Autodesk Inventor part; units mm, degrees
ref_plane "YZ Plane" through (0, 0, 0) normal (1, 0, 0) x (0, 1, 0)
ref_plane "XZ Plane" through (0, 0, 0) normal (0, 1, 0) x (-1, 0, 0)
ref_plane "XY Plane" through (0, 0, 0) normal (0, 0, 1) x (1, 0, 0)
sketch "Sketch1" plane through (0, 0, 0) normal (0, 0, 1) x (1, 0, 0)
  line L0 (0, 0) -> (30, 0) construction
  line L1 (30, 0) -> (30, 30) construction
  line L2 (30, 30) -> (0, 30) construction
  line L3 (0, 11.9722) -> (0, 0) construction
  circle A0 centre (0, 0) radius 30 construction
  circle A1 centre (30, 30) radius 30 construction
  circle A2 centre (30, 30) radius 35
  arc A3 (29.5798, 5.0035) -> (5.0035, 29.5798) centre (30, 30) ccw
  arc A4 (29.5798, 5.0035) -> (5.0035, 29.5798) centre (0, 0) ccw
  line L4 (30, 30) -> (0, 0) construction
  circle A5 centre (30, 30) radius 4
  circle A6 centre (8.7868, 8.7868) radius 3
  dimension "d3" = 60
  dimension "d4" = 70
  dimension "d0" = 30
  dimension "d1" = 30
  dimension "d2" = 60
  dimension "d5" = 50
  dimension "d6" = 8
  dimension "d7" = 6
extrude "Extrusion1" add sketch "Sketch1" along normal blind 5 contours A4 A3 | A6
extrude "Extrusion2" add sketch "Sketch1" against normal blind 5 contours A2 | A4 A3 | A6
properties part number "Geneva_driver"
The listing builds one solid part. Answer for the finished solid, in the listing's coordinates (mm). A direction names the side the tool comes from. Give positions to 0.01 mm unless a question says otherwise; leave off trailing zeros. Order: outer loops, then holes, each group sorted by start corner. A loop starts at its lowest first (then second) coordinate and runs counter-clockwise, first axis right, second up. Notation, with made-up numbers: (84, -9.5) - (141, -9.5) arc R20 ccw to (141, -2.5) - close; hole circle Ø1 at (60, 19). An arc over 180 degrees is marked (long way). Answer in a Markdown table with one row per item. Add a question column.
Q1. The part is cut by section A-A (z = -1). Determine the outline of the cut face in (x, y), then the cut area to 3 significant figures.
Q2. Find the intervals of material crossed by line 1 along Y through (x, z) = (30, -2); line 2 along Z through (x, y) = (11.5, 55.5); line 3 along Y through (x, z) = (30, 0.25), in increasing order. Write a range as [from, to].
Q3. Which of the six approach directions +Z, -Z, +X, -X, +Y, -Y give full straight-line access (tool end or side, diameter ignored) to faces 4 (the cylindrical face through (21.029, 21.396, 2.465)), 5 (the cylindrical face through (29.479, 26.034, -0.07))?
Q4. The part is cut by section C-C (y = 17). Determine the outline of the cut face in (x, z).
Q5. Given P1, Ø1, axis at x = 33.5, z = 0, coming from the +Y side; P2, Ø4, axis at x = 5.5, z = 1.5, coming from the +Y side; P3, Ø1.5, axis at x = 36.5, z = 0, coming from the -Y side; P4, Ø6.5, axis at x = 30, y = 30, coming from the +Z side, each flat-ended and moving along its own axis, determine where each tip first touches the part or whether it passes through.
Q6. For a pull along Y with two mould halves and no side action, classify faces 1 (the cylindrical face through (47.081, 48.255, 2.465)), 2 (the cylindrical face through (10.4, 6.257, 2.465)), 3 (the flat face through (9, 9, 5)) as released by +Y, released by -Y, zero draft, split by the parting line, or undercut.
Q7. The part is cut by section D-D (z = 3.5). Determine the outline of the cut face in (x, y), then the cut area to 3 significant figures.
Q8. The part is cut by section B-B (x = 10). Determine the outline of the cut face in (y, z), then the cut area to 3 significant figures.
Determined:
| question | item | result |
|---|---|---|
| 1 | outline | circle Ø70 at (30, 30); hole circle Ø8 at (30, 30) |
| 1 | area | 3,800 mm² |
| 2 | line 1 | y = [-5, 26], [34, 65] |
| 2 | line 2 | z = [-5, 0] |
| 2 | line 3 | y = [5, 26], [34, 55] |
| 3 | face 4 | +Z |
| 3 | face 5 | +Z, -Z |
| 4 | outline | (-2.5, -5) - (62.5, -5) - (62.5, 0) - (51.35, 0) - (51.35, 5) - (24.72, 5) - (24.72, 0) - (-2.5, 0) - close |
| 5 | P1 | stops at y = 64.87 |
| 5 | P2 | stops at y = 56.23 |
| 5 | P3 | stops at y = -4.52 |
| 5 | P4 | passes through |
| 6 | face 1 | split by the parting line |
| 6 | face 2 | undercut |
| 6 | face 3 | zero draft |
| 7 | outline | (5, 29.58) arc R30 cw to (29.58, 5) arc R25 ccw (long way) to start; circle Ø6 at (8.79, 8.79); hole circle Ø8 at (30, 30) |
| 7 | area | 1,640 mm² |
| 8 | outline | (1.28, -5) - (58.72, -5) - (58.72, 0) - (45, 0) - (45, 5) - (28.28, 5) - (28.28, 0) - (11.53, 0) - (11.53, 5) - (6.04, 5) - (6.04, 0) - (1.28, 0) - close |
| 8 | area | 398 mm² |
